Job drawing, mm, ordinate dimensions from the low corner. One solid piece. A direction names the side the tool comes from. Give positions to 0.01 mm unless a question says otherwise; leave off trailing zeros. Order: outer loops, then holes, each group sorted by start corner. A loop starts at its lowest first (then second) coordinate and runs counter-clockwise, first axis right, second up. Notation, with made-up numbers: (49, -39) - (93, -39) arc R29 cw to (93, -8) - close; hole circle Ø3 at (25, 22). An arc over 180 degrees is marked (long way). One line per item, written item: value.
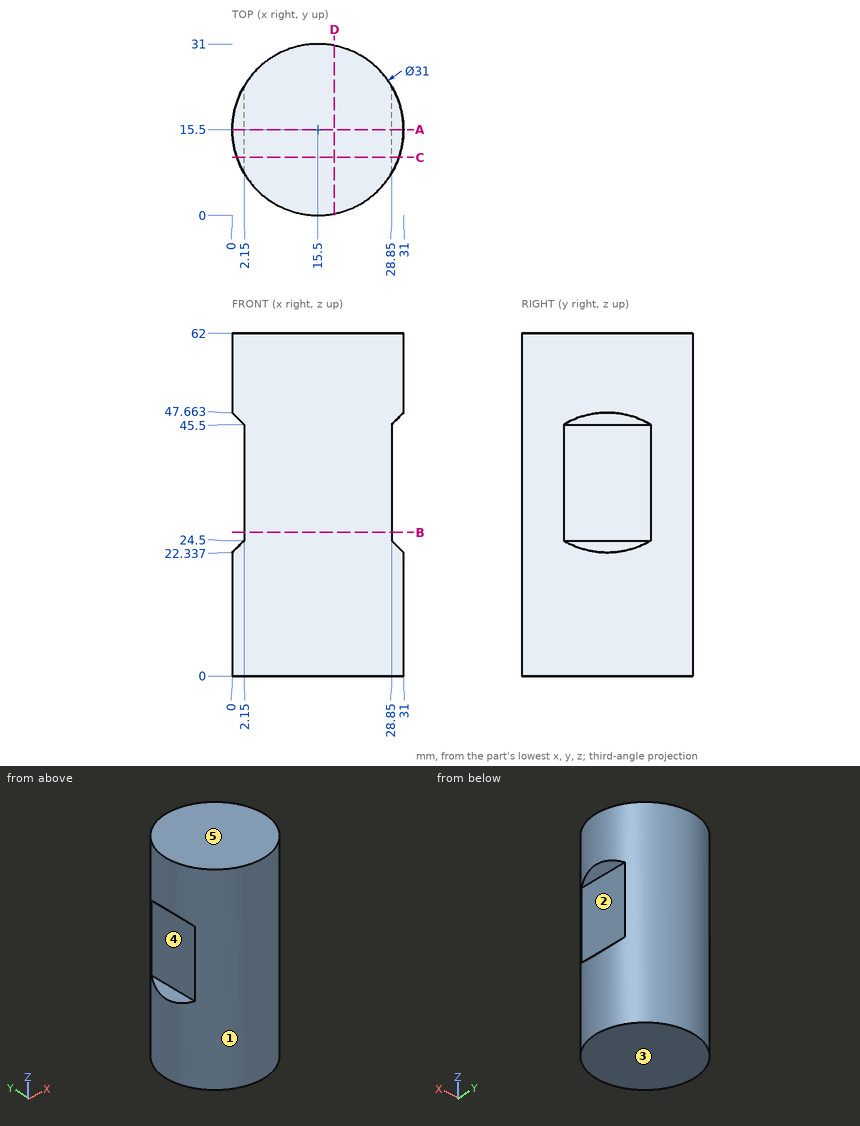
1) Wall check: line 1 along Y through (x, z) = (16, 56.5); line 2 along Z through (x, y) = (29.5, 12.5); line 3 along X through (y, z) = (15, 45). Give the ranges that are in metal, low to high. Write a range as [from, to].
Answer:
line 1: y = [0.01, 30.99]
line 2: z = [0, 23.85], [46.15, 62]
line 3: x = [2.15, 28.85]
2) Which spindle directions (+Z, -Z, +X, -X, +Y, -Y) get a long thin tool onto all of the face, cutting with end or side? Do the marked faces 1 and 2. Say none if no direction does.
Answer:
face 1: +Z, -Z
face 2: +X, +Y, -Y
3) Drop flat-ended pins along their axis: P1, Ø3, axis at x = 6.5, z = 45.5, coming from the +Y side (1 decimal); P2, Ø12, axis at y = 3, z = 48.5, coming from the +X side; P3, Ø4.5, axis at y = 18.5, z = 39, coming from the +X side. Give the stop position or say it passes through.
Answer:
P1: stops at y = 29.1
P2: stops at x = 29.57
P3: stops at x = 28.85
4) Two-plate mould, pull along Z, no slides. Class the marked faces 3, 4 and 5: pulls with the +Z half, pulls with the -Z half, needs draft (parallel to the pull), parting line crosses it, or undercut.
Answer:
face 3: pulls with the -Z half
face 4: undercut
face 5: pulls with the +Z half
5) Slice it at C-C on y = 10.5. Write the cut outline in (x, z), then the cut area to 3 significant figures.
Answer:
outline: (0.83, 0) - (30.17, 0) - (30.17, 23.17) - (28.85, 24.5) - (28.85, 45.5) - (30.17, 46.83) - (30.17, 62) - (0.83, 62) - (0.83, 46.83) - (2.15, 45.5) - (2.15, 24.5) - (0.83, 23.17) - close
area: 1,760 mm2
6) Slice it at D-D on x = 18.5. Write the cut outline in (y, z), then the cut area to 3 significant figures.
Answer:
outline: (0.29, 0) - (30.71, 0) - (30.71, 62) - (0.29, 62) - close
area: 1,890 mm2
7) Slice it at A-A on y = 15.5. Write the cut outline in (x, z).
Answer:
outline: (0, 0) - (31, 0) - (31, 22.34) - (28.85, 24.5) - (28.85, 45.5) - (31, 47.66) - (31, 62) - (0, 62) - (0, 47.66) - (2.15, 45.5) - (2.15, 24.5) - (0, 22.34) - close
8) Slice it at B-B on z = 26. Write the cut outline in (x, y).
Answer:
outline: (2.15, 7.62) arc R15.5 ccw to (28.85, 7.62) - (28.85, 23.38) arc R15.5 ccw to (2.15, 23.38) - close
